from build123d import *

# Parameters (mm, degrees)
BOSS_EXTRUDE2_DEPTH = 3
FILLET2_R           = 8
BOSS_EXTRUDE3_DEPTH = 44.7
SKETCH4_R           = 1.45
BOSS_EXTRUDE4_DEPTH = 6
SKETCH5_W           = 20.05
SKETCH5_H           = 7.70975521
SKETCH5_R           = 1.45
CUT_EXTRUDE2_DEPTH  = 3.3
BOSS_EXTRUDE5_REACH = 77.442
SKETCH7_W           = 10
SKETCH7_H           = 10
SKETCH7_R           = 1.525
CUT_EXTRUDE3_REACH  = 84.621
SKETCH8_W           = 28.937408921
SKETCH8_H           = 10
SKETCH11_R          = 1.525
SKETCH11_R_2        = 4.825
CUT_EXTRUDE4_DEPTH  = 3
SKETCH12_R          = 5.525
CUT_EXTRUDE5_DEPTH  = 0.5
SKETCH14_W          = 17.937492396
SKETCH14_H          = 5
CUT_EXTRUDE6_DEPTH  = 3


with BuildPart() as part:
    # Sketch2 → Boss-Extrude2 (new body)
    with BuildSketch(Plane(origin=(0, 0, 0), x_dir=(1, 0, 0), z_dir=(0, 1, 0))):
        Polygon((-53.10956872, -52.91705805), (-53.124237768, 1.36911662), (-19.174237768, 1.36911662), (-19.174237768, -52.91705805), align=None)
    extrude(amount=BOSS_EXTRUDE2_DEPTH)

    # Fillet2
    fillet2_edges = [part.edges().sort_by_distance(p)[0] for p in [
        (-53.10956872, 1.5, 52.91705805),
        (-53.124237768, 1.5, -1.36911662),
        (-19.174237768, 1.5, -1.36911662),
        (-19.174237768, 1.5, 52.91705805),
    ]]
    fillet(fillet2_edges, radius=FILLET2_R)

    # Sketch3 → Boss-Extrude3 (add)
    with BuildSketch(Plane(origin=(0, 3, 0), x_dir=(1, 0, 0), z_dir=(0, 1, 0))):
        with BuildLine():
            Line((-48.098156754, 4.70911662), (-24.198156754, 4.70911662))
            Line((-24.198156754, 4.70911662), (-24.198156754, 0.794945988))
            ThreePointArc((-24.198156754, 0.794945988), (-25.658756812, 1.224262543), (-27.174237768, 1.36911662))
            Line((-27.174237768, 1.36911662), (-45.12207574, 1.36911662))
            ThreePointArc((-45.12207574, 1.36911662), (-46.637556696, 1.224262543), (-48.098156754, 0.794945988))
            Line((-48.098156754, 0.794945988), (-48.098156754, 4.70911662))
        make_face()
    extrude(amount=-BOSS_EXTRUDE3_DEPTH)

    # Sketch4 → Boss-Extrude4 (add)
    with BuildSketch(Plane.XZ.offset(41.7)):
        with BuildLine():
            Line((-48.148156754, -1.125315107), (-48.148156754, -4.70911662))
            Line((-48.148156754, -4.70911662), (-24.148156754, -4.70911662))
            Line((-24.148156754, -4.70911662), (-24.148156754, -1.125315107))
            ThreePointArc((-24.148156754, -1.125315107), (-20.947846297, 1.245451192), (-19.298979621, 4.87088338))
            Line((-19.298979621, 4.87088338), (-52.997333887, 4.87088338))
            ThreePointArc((-52.997333887, 4.87088338), (-51.348467211, 1.245451192), (-48.148156754, -1.125315107))
        make_face()
        with Locations(Location((-41.048156754, 1.49088338, 0), (0, 0, 270))):
            Circle(SKETCH4_R, mode=Mode.SUBTRACT)
        with Locations(Location((-31.248156754, 1.49088338, 0), (0, 0, 270))):
            Circle(SKETCH4_R, mode=Mode.SUBTRACT)
    extrude(amount=-BOSS_EXTRUDE4_DEPTH)

    # Sketch5 → Cut-Extrude2 (cut)
    with BuildSketch(Plane.XZ.offset(41.7)):
        with Locations((-36.148152634, 1.016005775)):
            Rectangle(SKETCH5_W, SKETCH5_H)
        with Locations(Location((-31.248156754, 1.49088338, 0), (0, 0, 270))):
            Circle(SKETCH5_R, mode=Mode.SUBTRACT)
        with Locations(Location((-41.048156754, 1.49088338, 0), (0, 0, 270))):
            Circle(SKETCH5_R, mode=Mode.SUBTRACT)
    extrude(amount=-CUT_EXTRUDE2_DEPTH, mode=Mode.SUBTRACT)

    # Boss-Extrude5: up to this face of the body (flat: up to its plane)
    boss_extrude5_end = Plane(part.part.faces().sort_by_distance((-53.11690266, 1.5, 25.776132451))[0])
    # Sketch7 → Boss-Extrude5 (add, up to the picked face)
    with BuildSketch(Plane(origin=(-19.174237768, 0, 0), x_dir=(0, 0, -1), z_dir=(1, 0, 0)), mode=Mode.PRIVATE) as boss_extrude5_sk1:
        with Locations((-40.22705805, -2)):
            Rectangle(SKETCH7_W, SKETCH7_H)
        with Locations((-40.22705805, -2)):
            Circle(SKETCH7_R, mode=Mode.SUBTRACT)
    boss_extrude5_tool1 = split(extrude(boss_extrude5_sk1.sketch, amount=-BOSS_EXTRUDE5_REACH, mode=Mode.PRIVATE), bisect_by=boss_extrude5_end, keep=Keep.BOTH, mode=Mode.PRIVATE)
    add(boss_extrude5_tool1.solids().sort_by(Axis((-19.174238, 2.858579, 40.227058), (-1, 0, 0)))[0])

    # Cut-Extrude3: up to this face of the body (flat: up to its plane)
    cut_extrude3_end = Plane(part.part.faces().sort_by_distance((-36.146613335, 0, 17.301528841))[0])
    # Sketch8 → Cut-Extrude3 (cut, up to the picked face)
    with BuildSketch(Plane.XZ.offset(7), mode=Mode.PRIVATE) as cut_extrude3_sk1:
        with Locations((-36.142942229, 40.22705805)):
            Rectangle(SKETCH8_W, SKETCH8_H)
    cut_extrude3_tool1 = split(extrude(cut_extrude3_sk1.sketch, amount=-CUT_EXTRUDE3_REACH, mode=Mode.PRIVATE), bisect_by=cut_extrude3_end, keep=Keep.BOTH, mode=Mode.PRIVATE)
    add(cut_extrude3_tool1.solids().sort_by(Axis((-36.142942, -7, 40.227058), (0, 1, 0)))[0], mode=Mode.SUBTRACT)

    # Sketch11 → Cut-Extrude4 (cut)
    with BuildSketch(Plane.XZ):
        with Locations(Location((-45.644202791, 35.897058093, 0), (0, 0, 270))):
            Circle(SKETCH11_R)
        with Locations(Location((-26.644202791, 35.897058093, 0), (0, 0, 270))):
            Circle(SKETCH11_R)
        with Locations(Location((-36.144202791, 35.897058093, 0), (0, 0, 270))):
            Circle(SKETCH11_R_2)
    extrude(amount=-CUT_EXTRUDE4_DEPTH, mode=Mode.SUBTRACT)

    # Sketch12 → Cut-Extrude5 (cut)
    with BuildSketch(Plane.XZ):
        with Locations(Location((-36.144202791, 35.897058093, 0), (0, 0, 270))):
            Circle(SKETCH12_R)
    extrude(amount=-CUT_EXTRUDE5_DEPTH, mode=Mode.SUBTRACT)

    # Sketch14 → Cut-Extrude6 (cut)
    with BuildSketch(Plane(origin=(0, 3, 0), x_dir=(1, 0, 0), z_dir=(0, 1, 0))):
        with Locations((-36.142983966, -50.41705805)):
            Rectangle(SKETCH14_W, SKETCH14_H)
    extrude(amount=-CUT_EXTRUDE6_DEPTH, mode=Mode.SUBTRACT)


solid = part.part
Check sheet for the modelled part. Datum: model origin and axes. Units: mm. A direction names the side the tool comes from. Round coordinates to 2 decimals unless told otherwise and drop trailing zeros. Loops run counter-clockwise (first coordinate to the right, second up) from the corner with the lowest first, then second, coordinate; pieces in that order, holes last. Notation, with made-up numbers: M -39,83 L -4,83 A21 cw -4,96 Z; hole C 32,-9.75 d1. An arc over 180 degrees is marked long. One line per question, with ' | ' between items. Start each with the question number.
Item 1: Section check A-A (y = -2). Record the boundary of the cut face in (x, z).
Item 2: Release check for a two-part mould opening along Y. For faces 1 (the face through (-52, -7, 40)), 2 (the face through (-36, -40, -2.839)), 3 (the face through (-20.407, -1.542, 38.772)) record: released by +Y, released by -Y, zero draft, split by the parting line, or undercut.
Item 3: Set-up check for faces 4 (the face through (-26.123, -40, 1)), 5 (the face through (-34.48, 0.25, 30.63)), 6 (the face through (-45.112, 2, 50)): record each of +Z, -Z, +X, -X, +Y, -Y from which the full face is reachable in a straight line by a thin tool's end or side.
Item 4: Section check D-D (y = -31). Record the boundary of the cut face in (x, z).
Item 5: Section check B-B (z = 40). Record the boundary of the cut face in (x, y), and give its area (3 significant figures).
Item 6: Section check C-C (x = -35). Record the boundary of the cut face in (y, z), and give its area (3 significant figures).
Item 7: Gauge pin test, flat ends, axial feed: pin 1 Ø5.5 at (y, z) = (-3, 40.5) entering from -X; pin 2 Ø4 at (x, z) = (-31.25, 1.49) entering from -Y; pin 3 Ø3.5 at (y, z) = (1.5, 51.5) entering from -X; pin 4 Ø1.8 at (x, z) = (-26.64, 35.9) entering from -Y. Record the tip position at first contact, or that the pin passes through.
Item 8: Scan lines: probe 1 along Y at (x, z) = (-33, 24); probe 2 along Y at (x, z) = (-23.5, 1); probe 3 along Z at (x, y) = (-41, -7.5). Record each from-to range of solid material in increasing order.
Worked out:
1) outline: M -53.11,35.23 L -50.61,35.23 L -50.61,38.7 L -53.11,38.7 Z; M -53.11,41.75 L -50.61,41.75 L -50.61,45.23 L -53.11,45.23 Z; M -48.1,-4.71 L -24.2,-4.71 L -24.2,-0.79 A8 cw -27.17,-1.37 L -45.12,-1.37 A8 cw -48.1,-0.79 Z; M -21.67,35.23 L -19.17,35.23 L -19.17,38.7 L -21.67,38.7 Z; M -21.67,41.75 L -19.17,41.75 L -19.17,45.23 L -21.67,45.23 Z
2) face 1: released by -Y | face 2: zero draft | face 3: undercut
3) face 4: +Z, -Y | face 5: -Y | face 6: +Z, +Y, -Y
4) outline: M -48.1,-4.71 L -24.2,-4.71 L -24.2,-0.79 A8 cw -27.17,-1.37 L -45.12,-1.37 A8 cw -48.1,-0.79 Z
5) outline: M -53.11,-7 L -50.61,-7 L -50.61,-3.51 L -53.11,-3.51 Z; M -53.11,-0.49 L -50.61,-0.49 L -50.61,0 L -39.84,0 L -39.84,0.5 L -38.68,0.5 L -38.68,3 L -53.11,3 Z; M -33.61,0.5 L -32.44,0.5 L -32.44,0 L -21.67,0 L -21.67,-0.49 L -19.17,-0.49 L -19.17,3 L -33.61,3 Z; M -21.67,-7 L -19.17,-7 L -19.17,-3.51 L -21.67,-3.51 Z | area: 105 mm^2
6) outline: M -41.7,-4.71 L 3,-4.71 L 3,31.21 L 0.5,31.21 L 0.5,30.49 L 0,30.49 L 0,-1.37 L -35.7,-1.37 L -35.7,4.87 L -38.4,4.87 L -38.4,-2.84 L -41.7,-2.84 Z; M 0,41.3 L 0.5,41.3 L 0.5,40.58 L 3,40.58 L 3,47.92 L 0,47.92 Z | area: 280 mm^2
7) pin 1: x = -53.11 | pin 2: y = -38.4 | pin 3: x = -51.49 | pin 4: through
8) probe 1: 0 to 3 | probe 2: -41.7 to -35.7, 0 to 3 | probe 3: -4.71 to -1.37
